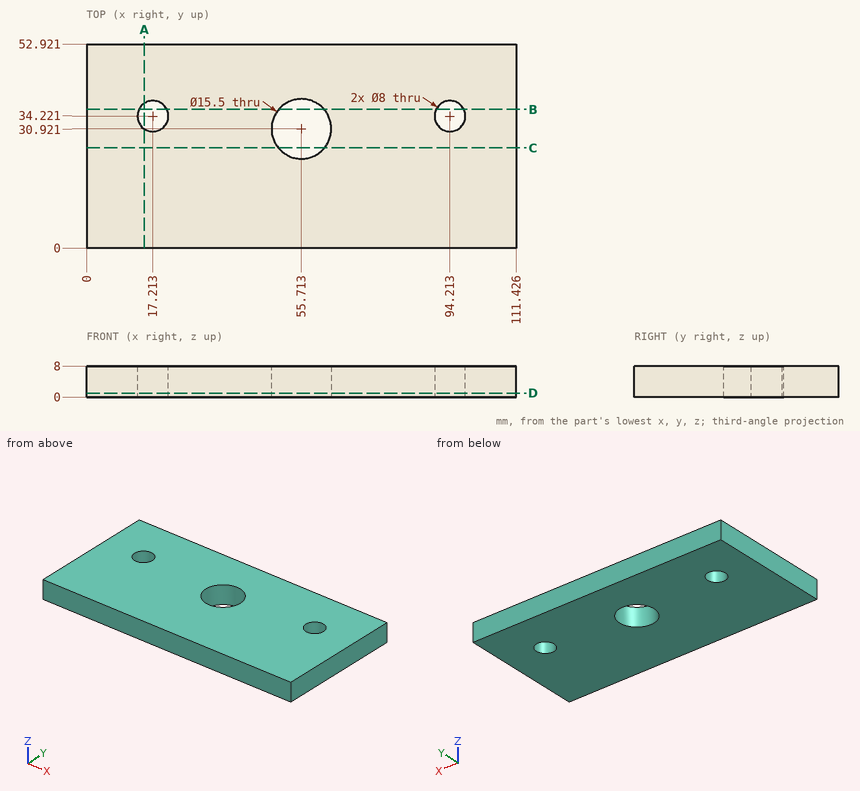
Here's the drawing with two shaded views (mm, measured from the low corner). I have some questions. Coordinates: 2 decimals unless noted, no trailing zeros. Order: outer loops, then holes, each group sorted by start corner. A loop starts at its lowest first (then second) coordinate and runs counter-clockwise, first axis right, second up.
Item 1: I need wall thicknesses on line 1 (Y direction, x = 92, z = 2.25); line 2 (Y direction, x = 54, z = 2); line 3 (X direction, y = 26.5, z = 5.75). Which ranges of each line are inside material? Lowest first, please.
Result sheet:
line 1: y = 0 to 30.89, 37.55 to 52.92
line 2: y = 0 to 23.36, 38.48 to 52.92
line 3: x = 0 to 49.35, 62.08 to 111.43
Item 2: If we section it at D-D on z = 1: List the corners of the cut face in (x, y) for me, plus the area to 3 significant figures.
Result sheet:
outline: (0, 0) - (111.43, 0) - (111.43, 52.92) - (0, 52.92) - close; hole circle Ø8 at (17.21, 34.22); hole circle Ø15.5 at (55.71, 30.92); hole circle Ø8 at (94.21, 34.22)
area: 5,610 mm2
Item 3: If we section it at A-A on x = 15: List the corners of the cut face in (y, z) for me.
Result sheet:
outline: (0, 0) - (30.89, 0) - (30.89, 8) - (0, 8) - close; (37.55, 0) - (52.92, 0) - (52.92, 8) - (37.55, 8) - close
Item 4: For P1, Ø9, axis at x = 94.21, y = 34.22, coming from the -Z side, with a flat end and sliding along its axis, tell me the tip position at first contact or that it passes through.
Result sheet:
P1: stops at z = 0
Item 5: If we section it at C-C on y = 26: List the corners of the cut face in (x, z) for me.
Result sheet:
outline: (0, 0) - (49.73, 0) - (49.73, 8) - (0, 8) - close; (61.7, 0) - (111.43, 0) - (111.43, 8) - (61.7, 8) - close
Item 6: If we section it at B-B on y = 36: List the corners of the cut face in (x, z) for me, plus the area to 3 significant figures.
Result sheet:
outline: (0, 0) - (13.63, 0) - (13.63, 8) - (0, 8) - close; (20.8, 0) - (49.86, 0) - (49.86, 8) - (20.8, 8) - close; (61.57, 0) - (90.63, 0) - (90.63, 8) - (61.57, 8) - close; (97.8, 0) - (111.43, 0) - (111.43, 8) - (97.8, 8) - close
area: 683 mm2
